Input: part model. Units: mm. Frame: model coordinates. Face numbers are marked on the shaded views. A direction names the side the tool comes from. Give positions to 0.01 mm unless a question says otherwise; leave off trailing zeros. Write each loop counter-clockwise with the first axis right and the second up, starting at its lowest first coordinate (ties: lowest second). Pieces come first, ordered by that corner, then holes. Notation, with made-up numbers: (64.5, 66.5) - (105.5, 66.5) arc R30 ccw to (105.5, 92.5) - close; hole circle Ø8 at (87.5, 72.25). An arc over 180 degrees is marked (long way). Answer as a JSON object with one key per item and string values. Group by question number.
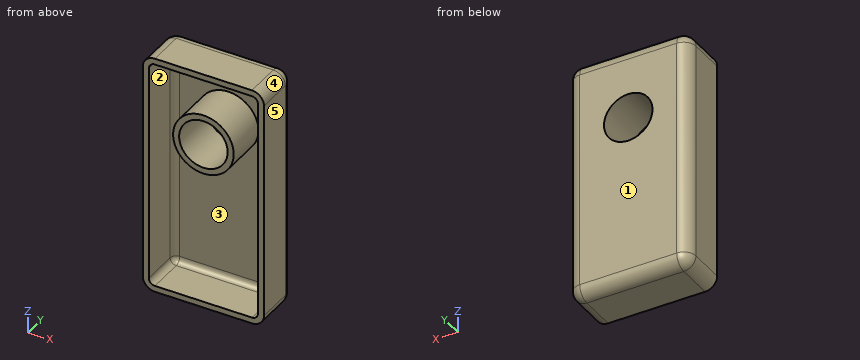
from build123d import *

# Parameters (mm, degrees)
F0_W     = 50
F0_H     = 100
F0_R     = 10
F1_DEPTH = 10
F2_R     = 5
F3_R     = 5
F4_T     = -2.5


with BuildPart() as f1:
    # F0 (on Front) → F1 (new body, symmetric)
    with BuildSketch(Plane.XZ):
        with Locations((0, 20)):
            Rectangle(F0_W, F0_H)
        Circle(F0_R, mode=Mode.SUBTRACT)
        with Locations((0, 40)):
            Circle(F0_R, mode=Mode.SUBTRACT)
        Circle(F0_R)
    extrude(amount=F1_DEPTH, both=True)

    # F2
    f2_edges = [f1.edges().sort_by_distance(p)[0] for p in [
        (-25, 0, 70),
        (25, 0, 70),
        (-25, 0, -30),
        (25, 0, -30),
    ]]
    fillet(f2_edges, radius=F2_R)

    # F3
    f3_edges = [f1.edges().sort_by_distance(p)[0] for p in [
        (0, 10, 70),
        (23.535534, 10, 68.535534),
        (25, 10, 20),
        (23.535534, 10, -28.535534),
        (0, 10, -30),
        (-23.535534, 10, -28.535534),
        (-25, 10, 20),
        (-23.535534, 10, 68.535534),
    ]]
    fillet(f3_edges, radius=F3_R)

    # F4
    f4_openings = [f1.faces().sort_by_distance(p)[0] for p in [
        (0, -10, 18.652943),
    ]]
    offset(amount=F4_T, openings=f4_openings)


solid = f1.part
1) Mould query, pull axis Z, two halves, no side actions, for the marked faces 3, 4 and 5. Classes: +Z half, -Z half, draft (parallel to the pull), parting line (faces both ways), or undercut.
2) Cut plane D-D on z = -1.5. Return the cut outline in (x, y), and give its area (3 significant figures).
3) Pin query (flat end, axial travel): P1, Ø8, axis at x = -0.5, z = 7, coming from the -Y side. Return the tip coordinate at first contact, or that it passes through.
4) Line query: line 1 along Z through (x, y) = (0, -0.75); line 2 along Z through (x, y) = (-15.5, 1); line 3 along X through (y, z) = (1, -19). Output: solid intervals per line, ascending. Write a range as from..to.
5) Cut plane C-C on x = 0. Return the cut outline in (y, z), and give its area (3 significant figures).
6) Reachability of the marked faces 1 and 2 from +Z, -Z, +X, -X, +Y, -Y: full face, straight path, thin tool, end or side. Return the list, or none.
7) Cut plane B-B on y = 0. Return the cut outline in (x, z).
8) Cut plane A-A on z = 40. Return the cut outline in (x, y).
Filled in:
{
 "1": {"face 3": "undercut", "face 4": "+Z half", "face 5": "draft"},
 "2": {"outline": "(-25, -10) - (-22.5, -10) - (-22.5, 5) arc R2.5 cw to (-20, 7.5) - (20, 7.5) arc R2.5 cw to (22.5, 5) - (22.5, -10) - (25, -10) - (25, 5) arc R5 ccw to (20, 10) - (-20, 10) arc R5 ccw to (-25, 5) - close", "area": "204 mm²"},
 "3": {"P1": "stops at y = 7.5"},
 "4": {"line 1": "z = -30..-27.5, 27.5..30, 50..52.5, 67.5..70", "line 2": "z = -30..-27.5, 67.5..70", "line 3": "x = -25..-22.5, 22.5..25"},
 "5": {"outline": "(-10, -30) - (5, -30) arc R5 ccw to (10, -25) - (10, 30) - (-10, 30) - (-10, 27.5) - (7.5, 27.5) - (7.5, -25) arc R2.5 cw to (5, -27.5) - (-10, -27.5) - close; (-10, 50) - (10, 50) - (10, 65) arc R5 ccw to (5, 70) - (-10, 70) - (-10, 67.5) - (5, 67.5) arc R2.5 cw to (7.5, 65) - (7.5, 52.5) - (-10, 52.5) - close", "area": "367 mm²"},
 "6": {"face 1": "+Z, -Z, +X, -X, +Y", "face 2": "-Y"},
 "7": {"outline": "(-25, -25) arc R5 ccw to (-20, -30) - (20, -30) arc R5 ccw to (25, -25) - (25, 65) arc R5 ccw to (20, 70) - (-20, 70) arc R5 ccw to (-25, 65) - close; circle Ø25 at (0, 40); hole (-22.5, -25) arc R2.5 ccw to (-20, -27.5) - (20, -27.5) arc R2.5 ccw to (22.5, -25) - (22.5, 65) arc R2.5 ccw to (20, 67.5) - (-20, 67.5) arc R2.5 ccw to (-22.5, 65) - close; hole circle Ø20 at (0, 40)"},
 "8": {"outline": "(-25, -10) - (-22.5, -10) - (-22.5, 5) arc R2.5 cw to (-20, 7.5) - (-12.5, 7.5) - (-12.5, -10) - (-10, -10) - (-10, 10) - (-20, 10) arc R5 ccw to (-25, 5) - close; (10, -10) - (12.5, -10) - (12.5, 7.5) - (20, 7.5) arc R2.5 cw to (22.5, 5) - (22.5, -10) - (25, -10) - (25, 5) arc R5 ccw to (20, 10) - (10, 10) - close"}
}
